CAD build for the part. Positions are in the model's coordinates, mm. Round coordinates to 2 decimals unless told otherwise and drop trailing zeros. Loops run counter-clockwise (first coordinate to the right, second up) from the corner with the lowest first, then second, coordinate; pieces in that order, holes last.
from build123d import *

# Parameters (mm, degrees)
SKETCH_1_R          = 2
SKETCH_1_R_2        = 1.5
EXTRUDE_1_DEPTH     = 2
SKETCH_2_W          = 80
SKETCH_2_H          = 23
CUT_EXTRUDE_1_DEPTH = 121.769408378
SKETCH_3_W          = 5
SKETCH_3_H          = 23
EXTRUDE_2_DEPTH     = 2
FILLET_1_R          = 2
FILLET_2_R          = 1
FILLET_3_R          = 2


with BuildPart() as part:
    # 草图1 → 凸台-拉伸1 (new body)
    with BuildSketch(Plane(origin=(0, 0, 0), x_dir=(1, 0, 0), z_dir=(0, 1, 0))):
        Polygon((55, 107.5), (55, 0), (-55, 0), (-55, 107.5), (-40, 107.5), (-40, 55), (40, 55), (40, 107.5), align=None)
        with Locations(Location((47.5, 32.5, 0), (0, 0, 270))):
            Circle(SKETCH_1_R, mode=Mode.SUBTRACT)
        with Locations(Location((47.5, 7.5, 0), (0, 0, 270))):
            Circle(SKETCH_1_R, mode=Mode.SUBTRACT)
        with Locations(Location((47.5, 79.5, 0), (0, 0, 270))):
            Circle(SKETCH_1_R, mode=Mode.SUBTRACT)
        with Locations(Location((47.5, 102.5, 0), (0, 0, 270))):
            Circle(SKETCH_1_R, mode=Mode.SUBTRACT)
        with Locations(Location((-47.5, 102.5, 0), (0, 0, 90))):
            Circle(SKETCH_1_R, mode=Mode.SUBTRACT)
        with Locations(Location((-47.5, 79.5, 0), (0, 0, 90))):
            Circle(SKETCH_1_R, mode=Mode.SUBTRACT)
        with Locations(Location((-47.5, 7.5, 0), (0, 0, 90))):
            Circle(SKETCH_1_R, mode=Mode.SUBTRACT)
        with Locations(Location((-47.5, 32.5, 0), (0, 0, 90))):
            Circle(SKETCH_1_R, mode=Mode.SUBTRACT)
        with Locations(Location((-32, 36, 0), (0, 0, 270))):
            Circle(SKETCH_1_R_2, mode=Mode.SUBTRACT)
        with Locations(Location((32, 36, 0), (0, 0, 90))):
            Circle(SKETCH_1_R_2, mode=Mode.SUBTRACT)
    extrude(amount=EXTRUDE_1_DEPTH)

    # 草图2 → 切除-拉伸1 (cut, through all)
    with BuildSketch(Plane(origin=(0, 2, 0), x_dir=(1, 0, 0), z_dir=(0, 1, 0))):
        with Locations((0, 19.5)):
            Rectangle(SKETCH_2_W, SKETCH_2_H)
        Polygon((-40, 49), (-25, 37), (-25, 49), align=None)
        Polygon((-20, 49), (-5, 49), (-20, 37), align=None)
        Polygon((0, 46.596875763), (-11.996094703, 37), (11.996094703, 37), align=None)
        Polygon((20, 37), (20, 49), (5, 49), align=None)
        Polygon((25, 49), (40, 49), (25, 37), align=None)
    extrude(amount=-CUT_EXTRUDE_1_DEPTH, mode=Mode.SUBTRACT)

    # 草图3 → 拉伸-薄壁2 (add)
    with BuildSketch(Plane(origin=(0, 2, 0), x_dir=(1, 0, 0), z_dir=(0, 1, 0))):
        Polygon((-40.690768562, 28.59732674), (39.309231438, 5.59732674), (40.690768562, 10.40267326), (-39.309231438, 33.40267326), align=None)
        Polygon((-39.309231438, 5.59732674), (40.690768562, 28.59732674), (39.309231438, 33.40267326), (-40.690768562, 10.40267326), align=None)
        with Locations((0, 19.5)):
            Rectangle(SKETCH_3_W, SKETCH_3_H)
    extrude(amount=-EXTRUDE_2_DEPTH)

    # 圆角1
    fillet_1_edges = [part.edges().sort_by_distance(p)[0] for p in [
        (55, 1, -107.5),
        (55, 1, 0),
        (-55, 1, 0),
        (-55, 1, -107.5),
        (-40, 1, -107.5),
        (-40, 1, -55),
        (40, 1, -55),
        (40, 1, -107.5),
    ]]
    fillet(fillet_1_edges, radius=FILLET_1_R)

    # 圆角2
    fillet_2_edges = [part.edges().sort_by_distance(p)[0] for p in [
        (-20, 1, -49),
        (-5, 1, -49),
        (-40, 1, -49),
        (-25, 1, -49),
        (-25, 1, -37),
        (25, 1, -37),
        (25, 1, -49),
        (40, 1, -49),
        (-30.952107056, 1, -8),
        (30.952107056, 1, -8),
        (30.952107056, 1, -31),
        (-30.952107056, 1, -31),
        (-9.047892944, 1, -19.5),
        (9.047892944, 1, -19.5),
        (2.5, 1, -31),
        (-2.5, 1, -31),
        (-2.5, 1, -8),
        (2.5, 1, -8),
        (11.996094703, 1, -37),
        (-11.996094703, 1, -37),
        (20, 1, -37),
        (5, 1, -49),
        (20, 1, -49),
        (-20, 1, -37),
    ]]
    fillet(fillet_2_edges, radius=FILLET_2_R)

    # 圆角3
    fillet_3_edges = [part.edges().sort_by_distance(p)[0] for p in [
        (40, 1, -28.398730779),
        (40, 1, -10.601269221),
        (-40, 1, -10.601269221),
        (-40, 1, -28.398730779),
        (-2.5, 1, -22.820019221),
        (2.5, 1, -16.179980779),
        (2.5, 1, -22.820019221),
        (-2.5, 1, -16.179980779),
        (0, 1, -46.596875763),
    ]]
    fillet(fillet_3_edges, radius=FILLET_3_R)


solid = part.part
Item 1: Flat gauge pin, fed straight in: P1, Ø1, axis at x = 9.5, y = 1, coming from the -Z side. Where does the tip first touch, or does it go through?
Verdict:
P1: stops at z = -55
Item 2: Cut at C-C (x = 32). List the corners of the cut face in (y, z), plus the area to 3 significant figures.
Verdict:
outline: (0, -55) - (2, -55) - (2, -49) - (0, -49) - close; (0, -42.6) - (2, -42.6) - (2, -37.5) - (0, -37.5) - close; (0, -34.5) - (2, -34.5) - (2, -26.1) - (0, -26.1) - close; (0, -12.9) - (2, -12.9) - (2, 0) - (0, 0) - close
area: 64.8 mm2
Item 3: Mould opens along X. For faces 1 (the flat face through (-12.723, 1.014, -42.822)), 2 (the flat face through (-24.7, 1, -15)) say: released by +X, released by -X, zero draft, split by the parting line, or undercut.
Verdict:
face 1: undercut
face 2: undercut
Item 4: Wall check: L1, parallel to X at y = 0.95, z = -36; L2, parallel to X at y = 1.6, z = -7.5; L3, parallel to X at y = 1.1, z = -79.5. Give the ranges that are in metal, low to high.
Verdict:
L1: x = -55 to -33.5, -30.5 to 30.5, 33.5 to 55
L2: x = -55 to -49.5, -45.5 to 45.5, 49.5 to 55
L3: x = -55 to -49.5, -45.5 to -40, 40 to 45.5, 49.5 to 55
Item 5: Cut at B-B (z = -79.5). List the corners of the cut face in (x, y), plus the area to 3 significant figures.
Verdict:
outline: (-55, 0) - (-49.5, 0) - (-49.5, 2) - (-55, 2) - close; (-45.5, 0) - (-40, 0) - (-40, 2) - (-45.5, 2) - close; (40, 0) - (45.5, 0) - (45.5, 2) - (40, 2) - close; (49.5, 0) - (55, 0) - (55, 2) - (49.5, 2) - close
area: 44.0 mm2
Item 6: Cut at D-D (y = 1.1). State how many separate pieces and enclosed holes the cut face has, plus the area to 3 significant figures.
Verdict:
separate pieces: 1
enclosed holes: 21
area: 6,070 mm2
Item 7: Cut at A-A (x = 47.5). List the corners of the cut face in (y, z).
Verdict:
outline: (0, -107.5) - (2, -107.5) - (2, -104.5) - (0, -104.5) - close; (0, -100.5) - (2, -100.5) - (2, -81.5) - (0, -81.5) - close; (0, -77.5) - (2, -77.5) - (2, -34.5) - (0, -34.5) - close; (0, -30.5) - (2, -30.5) - (2, -9.5) - (0, -9.5) - close; (0, -5.5) - (2, -5.5) - (2, 0) - (0, 0) - close
